from build123d import *

# Parameters (mm, degrees)
SKETCH1_W                = 64
SKETCH1_H                = 22
BOSS_EXTRUDE1_DEPTH      = 4
BOSS_EXTRUDE1_DEPTH_BACK = 17
SKETCH2_W                = 10
SKETCH2_H                = 12
CUT_EXTRUDE1_DEPTH       = 5
SKETCH3_R                = 1
CUT_EXTRUDE2_DEPTH       = 7
SKETCH4_R                = 5
CUT_EXTRUDE3_DEPTH       = 21
CUT_EXTRUDE4_START       = -17
SKETCH7_W                = 22.400000327
SKETCH7_H                = 12.400000179
CUT_EXTRUDE4_DEPTH       = 17
CUT_EXTRUDE5_REACH       = 9
SKETCH8_W                = 1
SKETCH8_H                = 4
CUT_EXTRUDE7_DEPTH       = 21
SKETCH9_R                = 8
CUT_EXTRUDE6_DEPTH       = 3


with BuildPart() as part:
    # Sketch1 → Boss-Extrude1 (new body, two sides)
    with BuildSketch(Plane(origin=(54.112238255, 0, 0), x_dir=(0, 0, -1), z_dir=(1, 0, 0))) as boss_extrude1_sk:
        with Locations((44.500000075, 65.042436513)):
            Rectangle(SKETCH1_W, SKETCH1_H)
    extrude(amount=BOSS_EXTRUDE1_DEPTH)
    extrude(boss_extrude1_sk.sketch, amount=-BOSS_EXTRUDE1_DEPTH_BACK)

    # Sketch2 → Cut-Extrude1 (cut)
    with BuildSketch(Plane.XY.offset(-12.500000075)):
        with Locations((49.112238255, 65.042436513)):
            Rectangle(SKETCH2_W, SKETCH2_H)
    extrude(amount=-CUT_EXTRUDE1_DEPTH, mode=Mode.SUBTRACT)

    # Sketch3 → Cut-Extrude2 (cut)
    with BuildSketch(Plane.ZY.offset(-37.112238255)):
        with Locations((-14.499999836, 65.042436513)):
            Circle(SKETCH3_R)
        with Locations((-42.500000313, 65.042436513)):
            Circle(SKETCH3_R)
    extrude(amount=-CUT_EXTRUDE2_DEPTH, mode=Mode.SUBTRACT)

    # Sketch4 → Cut-Extrude3 (cut)
    with BuildSketch(Plane.ZY.offset(-37.112238255)):
        with Locations((-66.500000075, 65.042436513)):
            Circle(SKETCH4_R)
    extrude(amount=-CUT_EXTRUDE3_DEPTH, mode=Mode.SUBTRACT)

    # Sketch7 → Cut-Extrude4 (cut)
    with BuildSketch(Plane.ZY.offset(-37.112238255).offset(CUT_EXTRUDE4_START)):
        with Locations((-28.500000075, 65.042436514)):
            Rectangle(SKETCH7_W, SKETCH7_H)
    extrude(amount=CUT_EXTRUDE4_DEPTH, mode=Mode.SUBTRACT)

    # Sketch8 → Cut-Extrude5 (cut, up to next)
    with BuildSketch(Plane(origin=(44.112238255, 0, 0), x_dir=(0, 0, -1), z_dir=(1, 0, 0)), mode=Mode.PRIVATE) as cut_extrude5_sk1:
        with Locations((16.799999911, 65.042436513)):
            Rectangle(SKETCH8_W, SKETCH8_H)
    cut_extrude5_tool1 = extrude(cut_extrude5_sk1.sketch, amount=-CUT_EXTRUDE5_REACH, mode=Mode.PRIVATE) & part.part
    add(cut_extrude5_tool1.solids().sort_by_distance((44.112238, 65.042437, -16.8))[0], mode=Mode.SUBTRACT)

    # Sketch10 → Cut-Extrude7 (cut)
    with BuildSketch(Plane(origin=(58.112238255, 0, 0), x_dir=(0, 0, -1), z_dir=(1, 0, 0))):
        with BuildLine():
            ThreePointArc((12.500000075, 71.042436513), (13.964466169, 74.577970419), (17.500000075, 76.042436513))
            Line((17.500000075, 76.042436513), (12.500000075, 76.042436513))
            Line((12.500000075, 76.042436513), (12.500000075, 71.042436513))
        make_face()
        with BuildLine():
            ThreePointArc((71.500000075, 76.042436513), (75.03553398, 74.577970419), (76.500000075, 71.042436513))
            Line((76.500000075, 71.042436513), (76.500000075, 76.042436513))
            Line((76.500000075, 76.042436513), (71.500000075, 76.042436513))
        make_face()
        with BuildLine():
            Line((76.500000075, 54.042436513), (76.500000075, 59.042436513))
            ThreePointArc((76.500000075, 59.042436513), (75.03553398, 55.506902607), (71.500000075, 54.042436513))
            Line((71.500000075, 54.042436513), (76.500000075, 54.042436513))
        make_face()
        with BuildLine():
            Line((12.500000075, 54.042436513), (17.500000075, 54.042436513))
            ThreePointArc((17.500000075, 54.042436513), (13.964466169, 55.506902607), (12.500000075, 59.042436513))
            Line((12.500000075, 59.042436513), (12.500000075, 54.042436513))
        make_face()
    extrude(amount=-CUT_EXTRUDE7_DEPTH, mode=Mode.SUBTRACT)

    # Sketch9 → Cut-Extrude6 (cut)
    with BuildSketch(Plane(origin=(58.112238255, 0, 0), x_dir=(0, 0, -1), z_dir=(1, 0, 0))):
        with Locations((66.500000075, 65.042436513)):
            Circle(SKETCH9_R)
    extrude(amount=-CUT_EXTRUDE6_DEPTH, mode=Mode.SUBTRACT)


solid = part.part
The model under review builds one solid part; all positions refer to its coordinate system, in mm. A direction names the side the tool comes from. Coordinates: 2 decimals unless noted, no trailing zeros. Loops run counter-clockwise (first coordinate to the right, second up) from the corner with the lowest first, then second, coordinate; pieces in that order, holes last.
(1) Draft analysis for pull direction Y (two halves, no side actions). For faces 4 (the flat face through (48, 76.042, -44)), 5 (the flat face through (44.112, 65, -43)), 6 (the flat face through (41, 65, -12.5)), state which applies: +Y half, -Y half, draft (parallel to the pull), parting line (faces both ways), or undercut.
Determined:
face 4: +Y half
face 5: undercut
face 6: draft
(2) Consider section D-D, the plane z = -24.5. Give the boundary of the cut face in (x, y), plus the area to 3 significant figures.
Determined:
outline: (37.11, 54.04) - (58.11, 54.04) - (58.11, 76.04) - (37.11, 76.04) - (37.11, 71.24) - (54.11, 71.24) - (54.11, 58.84) - (37.11, 58.84) - close
area: 251 mm2
(3) Wall thickness on L1, parallel to Y at x = 57.4, z = -66.5; L2, parallel to Z at x = 39.5, y = 65.5; L3, parallel to Y at x = 38.75, z = -23.5: over which ranges is each line inside the solid? List them lowest first.
Determined:
L1: y = 54.04 to 57.04, 73.04 to 76.04
L2: z = -76.5 to -71.48, -61.52 to -43.39, -41.61 to -39.7, -16.3 to -15.39, -13.61 to -12.5
L3: y = 54.04 to 58.84, 71.24 to 76.04
(4) Consider section A-A, the plane z = -66.5. Give the boundary of the cut face in (x, y), plus the area to 3 significant figures.
Determined:
outline: (37.11, 54.04) - (58.11, 54.04) - (58.11, 57.04) - (55.11, 57.04) - (55.11, 60.04) - (37.11, 60.04) - close; (37.11, 70.04) - (55.11, 70.04) - (55.11, 73.04) - (58.11, 73.04) - (58.11, 76.04) - (37.11, 76.04) - close
area: 234 mm2
(5) Consider section B-B, the plane x = 49. Give the boundary of the cut face in (y, z), plus the area to 3 significant figures.
Determined:
outline: (54.04, -71.5) arc R5 ccw to (59.04, -76.5) - (71.04, -76.5) arc R5 ccw to (76.04, -71.5) - (76.04, -17.5) arc R5 ccw to (71.04, -12.5) - (71.04, -17.3) - (71.24, -17.3) - (71.24, -39.7) - (58.84, -39.7) - (58.84, -17.3) - (59.04, -17.3) - (59.04, -12.5) arc R5 ccw to (54.04, -17.5) - close; hole circle Ø10 at (65.04, -66.5)
area: 973 mm2
(6) Consider section C-C, the plane y = 68. Give the boundary of the cut face in (x, z), plus the area to 3 significant figures.
Determined:
outline: (37.11, -76.5) - (58.11, -76.5) - (58.11, -73.93) - (55.11, -73.93) - (55.11, -70.53) - (37.11, -70.53) - close; (37.11, -62.47) - (55.11, -62.47) - (55.11, -59.07) - (58.11, -59.07) - (58.11, -12.5) - (54.11, -12.5) - (54.11, -39.7) - (37.11, -39.7) - close; (37.11, -17.3) - (44.11, -17.3) - (44.11, -12.5) - (37.11, -12.5) - close
area: 725 mm2
(7) Insertion check: P1, Ø2, axis at y = 65.5, z = -35, coming from the -X side; P2, Ø1.4, axis at x = 47, z = -14.5, coming from the +Y side; P3, Ø0.5, axis at x = 41, z = -17, coming from the +Y side. Each pin has a flat end and moves straight along its axis. Give the tip position at first contact, or say it passes through.
Determined:
P1: stops at x = 54.11
P2: stops at y = 75.48
P3: stops at y = 76.04
(8) Tool access review of faces 1 (the flat face through (49, 59.042, -15)), 2 (the flat face through (46, 65, -39.7)), 3 (the cylindrical face through (56.63, 67.45, -74.13)): name each direction out of +Z, -Z, +X, -X, +Y, -Y from which nothing blocks a thin tool from reaching the whole face with its end or side.
Determined:
face 1: +Z
face 2: -X
face 3: +X
